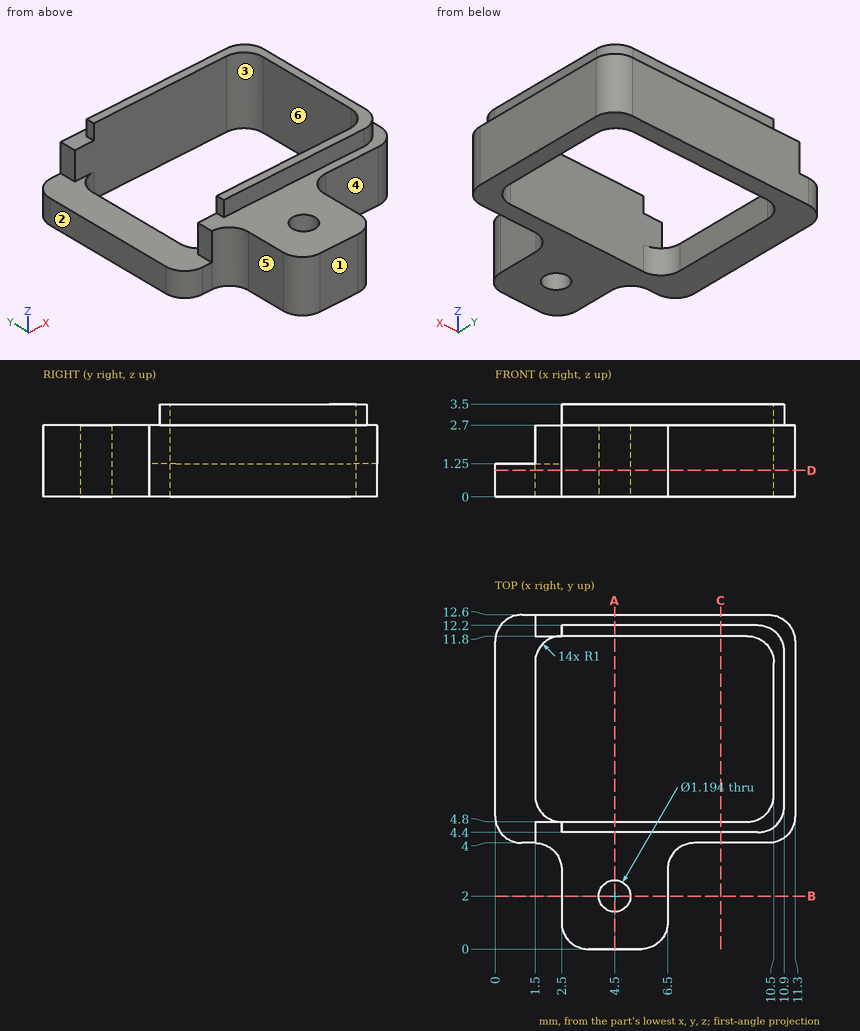
Study the drawing (mm; zero at the part's minimum x, y, z) and answer. A direction names the side the tool comes from. Give positions to 0.01 mm unless a question says otherwise; leave off trailing zeros. Write each loop counter-clockwise with the first axis right and the second up, starting at its lowest first coordinate (ties: lowest second). Pieces come first, ordered by that corner, then holes.
Item 1: Flat-ended cylindrical pins translate along their axes: P1, Ø1, axis at x = 4.5, y = 2, coming from the +Z side; P2, Ø3, axis at x = 1, y = 7, coming from the +Z side; P3, Ø1.5, axis at y = 7, z = 3, coming from the +X side; P4, Ø1.4, axis at x = 9, z = 1.5, coming from the -Y side. Find the tip coordinate at first contact, or state that the pin passes through.
Item 2: Section C-C, the plane x = 8.5 is taken. Write down the section's boundary in (y, z).
Item 3: Section A-A, the plane x = 4.5 is taken. Write down the section's boundary in (y, z), plus the area to 3 significant figures.
Item 4: Determine the mould class of the marked faces 1, 2 and 3 for opening direction X: released by +X, released by -X, zero draft, split by the parting line, or undercut.
Item 5: Section D-D, the plane z = 1 is taken. Write down the section's boundary in (x, y).
Item 6: Section B-B, the plane y = 2 is taken. Write down the section's boundary in (x, z).
Item 7: Which of the six approach directions +Z, -Z, +X, -X, +Y, -Y give full straight-line access (tool end or side, diameter ignored) to the marked faces 4, 5 and 6?
Item 8: Find the intervals of material crossed by line 1 along Y through (x, z) = (4.5, 0.8); line 2 along Y through (x, z) = (6.25, 2.85); line 3 along Y through (x, z) = (3.75, 2.15), in increasing order.
Completed:
1. P1: passes through
1. P2: stops at z = 1.25
1. P3: stops at x = 11.3
1. P4: stops at y = 4
2. outline: (4, 0) - (4.8, 0) - (4.8, 3.5) - (4.4, 3.5) - (4.4, 2.7) - (4, 2.7) - close; (11.8, 0) - (12.6, 0) - (12.6, 2.7) - (12.2, 2.7) - (12.2, 3.5) - (11.8, 3.5) - close
3. outline: (0, 0) - (1.4, 0) - (1.4, 2.7) - (0, 2.7) - close; (2.6, 0) - (4.8, 0) - (4.8, 3.5) - (4.4, 3.5) - (4.4, 2.7) - (2.6, 2.7) - close; (11.8, 0) - (12.6, 0) - (12.6, 2.7) - (12.2, 2.7) - (12.2, 3.5) - (11.8, 3.5) - close
3. area: 12.5 mm2
4. face 1: zero draft
4. face 2: released by -X
4. face 3: undercut
5. outline: (0, 5) arc R1 ccw to (1, 4) - (1.5, 4) arc R1 cw to (2.5, 3) - (2.5, 1) arc R1 ccw to (3.5, 0) - (5.5, 0) arc R1 ccw to (6.5, 1) - (6.5, 3) arc R1 cw to (7.5, 4) - (10.3, 4) arc R1 ccw to (11.3, 5) - (11.3, 11.6) arc R1 ccw to (10.3, 12.6) - (1, 12.6) arc R1 ccw to (0, 11.6) - close; hole (1.5, 5.8) arc R1 ccw to (2.5, 4.8) - (9.5, 4.8) arc R1 ccw to (10.5, 5.8) - (10.5, 10.8) arc R1 ccw to (9.5, 11.8) - (2.5, 11.8) arc R1 ccw to (1.5, 10.8) - close; hole circle Ø1.19 at (4.5, 2)
6. outline: (2.5, 0) - (3.9, 0) - (3.9, 2.7) - (2.5, 2.7) - close; (5.1, 0) - (6.5, 0) - (6.5, 2.7) - (5.1, 2.7) - close
7. face 4: +Z, -Z, +X, -Y
7. face 5: +Z, -Z, -X, -Y
7. face 6: +Z, -Z
8. line 1: y = 0 to 1.4, 2.6 to 4.8, 11.8 to 12.6
8. line 2: y = 4.4 to 4.8, 11.8 to 12.2
8. line 3: y = 0 to 4.8, 11.8 to 12.6
